```python
from build123d import *
from build123d.topology import SkipClean

# Parameters (mm, degrees)
EXTRUDE1_DEPTH               = 0.000254
SKETCH8_R                    = 2.413
EXTRUDE8_DEPTH               = 7.62
SKETCH6_R                    = 5.715
EXTRUDE6_DEPTH               = 2.413
SKETCH4_R                    = 0.254
EXTRUDE4_DEPTH               = 6.731
SKETCH5_R                    = 1.0033
EXTRUDE5_DEPTH               = 12.954
FILLET2_R                    = 0.889
CHAMFER1_SIZE                = 0.635
CHAMFER3_SIZE                = 0.635
EXTRUDE9_DEPTH               = 12.954
EXTRUDE11_DEPTH              = 6.731
CIRPATTERN1_COUNT            = 8
EXTRUDE12_DEPTH              = 6.731
CHAMFER4_SIZE                = 0.381
CHAMFER4_SIZE2               = 0.659911358
EXTRUDE13_DEPTH              = 0.6604
CUT_REVOLVE1_ANGLE           = 130
CUT_REVOLVE1_OTHER_WAY_ANGLE = 90
BOSS_EXTRUDE1_DEPTH          = 6.071088642
CUT_EXTRUDE1_DEPTH           = 0.838688642
CHAMFER5_SIZE                = 0.1016
CHAMFER6_SIZE                = 0.3048
SKETCH27_R                   = 0.381
CUT_EXTRUDE5_DEPTH           = 16.268548261
CUT_EXTRUDE7_DEPTH           = 1.27
SKETCH29_R                   = 0.6604
BOSS_EXTRUDE2_DEPTH          = 1.016
BOSS_EXTRUDE3_START          = -0.762
SKETCH30_R                   = 1.0033
BOSS_EXTRUDE3_DEPTH          = 0.762


with BuildPart() as part:
    # Sketch1 → Extrude1 (new body)
    with BuildSketch(Plane.XY):
        with BuildLine():
            Line((-1.242889362, 3.556), (-1.813523477, 0.319773119))
            ThreePointArc((-1.813523477, 0.319773119), (0, -1.8415), (1.813523477, 0.319773119))
            Line((1.813523477, 0.319773119), (1.242889362, 3.556))
            Line((1.242889362, 3.556), (-1.242889362, 3.556))
        make_face()
    extrude(amount=EXTRUDE1_DEPTH)

    # Sketch8 → Extrude8 (add)
    with BuildSketch(Plane.XY.offset(0.000254)):
        with Locations(Location((0, 0, 0), (0, 0, 129.743387424))):
            Circle(SKETCH8_R)
    extrude(amount=EXTRUDE8_DEPTH)

    # Sketch6 → Extrude6 (add)
    with BuildSketch(Plane.XY.offset(0.000254)):
        Circle(SKETCH6_R)
    extrude(amount=EXTRUDE6_DEPTH)

    # Sketch4 → Extrude4 (cut)
    with BuildSketch(Plane.XY.offset(7.620254)):
        Circle(SKETCH4_R)
    extrude(amount=-EXTRUDE4_DEPTH, mode=Mode.SUBTRACT)

    # Sketch5 → Extrude5 (add)
    with BuildSketch(Plane(origin=(0, 0, 0), x_dir=(-1, 0, 0), z_dir=(0, 0, -1))):
        with Locations(Location((0, 0, 0), (0, 0, 180))):
            Circle(SKETCH5_R)
    extrude(amount=EXTRUDE5_DEPTH)

    # Fillet2
    fillet2_edges = [part.edges().sort_by_distance(p)[0] for p in [
        (1.242889362, 3.556, 0.000127),
        (-1.242889362, 3.556, 0.000127),
    ]]
    fillet(fillet2_edges, radius=FILLET2_R)

    # Chamfer1
    chamfer1_edges = [part.edges().sort_by_distance(p)[0] for p in [
        (-5.715, 0, 0.000254),
    ]]
    chamfer(chamfer1_edges, length=CHAMFER1_SIZE)

    # Chamfer3
    chamfer3_edges = [part.edges().sort_by_distance(p)[0] for p in [
        (-5.715, 0, 2.413254),
    ]]
    chamfer(chamfer3_edges, length=CHAMFER3_SIZE)

    # Sketch9 → Extrude9 (add)
    with BuildSketch(Plane(origin=(0, 0, 0), x_dir=(-1, 0, 0), z_dir=(0, 0, -1))):
        with BuildLine():
            Line((-0.3175, 3.302), (0.3175, 3.302))
            ThreePointArc((0.3175, 3.302), (0.586907684, 3.190407684), (0.6985, 2.921))
            Line((0.6985, 2.921), (0.6985, 0))
            Line((0.6985, 0), (-0.6985, 0))
            Line((-0.6985, 0), (-0.6985, 2.921))
            ThreePointArc((-0.6985, 2.921), (-0.586907684, 3.190407684), (-0.3175, 3.302))
        make_face()
    extrude(amount=EXTRUDE9_DEPTH)

    # Sketch17 → Extrude11 (cut)
    with BuildSketch(Plane.XY.offset(7.620254)):
        with BuildLine():
            Line((0, 0), (0, 0.8128))
            ThreePointArc((0, 0.8128), (0.077181384, 0.80912723), (0.153665255, 0.798142111))
            ThreePointArc((0.153665255, 0.798142111), (0.281884616, 0.680529664), (0.455713955, 0.673029443))
            ThreePointArc((0.455713955, 0.673029443), (0.517563871, 0.626714831), (0.574736392, 0.574736392))
            Line((0.574736392, 0.574736392), (0, 0))
        make_face()
    extrude11 = extrude(amount=-EXTRUDE11_DEPTH, mode=Mode.SUBTRACT)

    # CirPattern1: Extrude11 ×8 about axis
    cirpattern1_axis = Axis((0, 0, 0), (0, 0, 1))
    for i in range(1, CIRPATTERN1_COUNT):
        add(extrude11.rotate(cirpattern1_axis, i * 360 / CIRPATTERN1_COUNT), mode=Mode.SUBTRACT)

    # Sketch18 → Extrude12 (add)
    with BuildSketch(Plane.XY.offset(7.620254)):
        Polygon((-0.539167209, 0.608229037), (0.811331666, 0.048834087), (0.986294531, 0.471231809), (-0.364204343, 1.030626759), align=None)
    extrude(amount=-EXTRUDE12_DEPTH)

    # Chamfer4
    chamfer4_edges = [part.edges().sort_by_distance(p)[0] for p in [
        (0.136082229, 0.328531562, 7.620254),
    ]]
    chamfer4_side = [part.faces().sort_by_distance(p)[0] for p in [
        (1.499116567, -1.802914954, 7.620254),
    ]]
    chamfer(chamfer4_edges, length=CHAMFER4_SIZE, length2=CHAMFER4_SIZE2, reference=chamfer4_side[0])

    # Sketch19 → Extrude13 (cut)
    with SkipClean():  # the faces are left unmerged after this step: merging them gives an invalid solid
        with BuildSketch(Plane.XY.offset(7.620254)):
            with BuildLine():
                Line((0.811331666, 0.048834087), (-0.539167209, 0.608229037))
                ThreePointArc((-0.539167209, 0.608229037), (-0.311045094, -0.750929284), (0.811331666, 0.048834087))
            make_face()
        extrude(amount=-EXTRUDE13_DEPTH, mode=Mode.SUBTRACT)

    # Sketch20 → Cut-Revolve1 (revolve, cut)
    with SkipClean():  # the faces are left unmerged after this step: merging them gives an invalid solid
        with BuildSketch(Plane(origin=(0, 0, 0), x_dir=(0, 0, -1), z_dir=(1, 0, 0))):
            Polygon((-6.959854, -0.8128), (-6.959854, 0), (-6.147054, 0), align=None)
        revolve(axis=Axis((0, 0, 7.389643883), (0, 0, -1)), revolution_arc=CUT_REVOLVE1_ANGLE, mode=Mode.SUBTRACT)

    # Sketch20 → Cut-Revolve1 other way (revolve, cut)
    with SkipClean():  # the faces are left unmerged after this step: merging them gives an invalid solid
        with BuildSketch(Plane(origin=(0, 0, 0), x_dir=(0, 0, -1), z_dir=(1, 0, 0))):
            Polygon((-6.959854, -0.8128), (-6.959854, 0), (-6.147054, 0), align=None)
        revolve(axis=Axis((0, 0, 7.389643883), (0, 0, 1)), revolution_arc=CUT_REVOLVE1_OTHER_WAY_ANGLE, mode=Mode.SUBTRACT)

    # Sketch21 → Boss-Extrude1 (add)
    with SkipClean():  # the faces are left unmerged after this step: merging them gives an invalid solid
        with BuildSketch(Plane.XY.offset(6.960342642)):
            with BuildLine():
                Line((-0.459893976, 0.575392988), (-0.539167209, 0.608229037))
                ThreePointArc((-0.539167209, 0.608229037), (-0.311045094, -0.750929284), (0.811331666, 0.048834087))
                Line((0.811331666, 0.048834087), (0.732058433, 0.081670135))
                ThreePointArc((0.732058433, 0.081670135), (-0.281884616, -0.680529664), (-0.459893976, 0.575392988))
            make_face()
        extrude(amount=-BOSS_EXTRUDE1_DEPTH)

    # Sketch22 → Cut-Extrude1 (cut)
    with SkipClean():  # the faces are left unmerged after this step: merging them gives an invalid solid
        with BuildSketch(Plane.XY.offset(6.960342642)):
            with BuildLine():
                Line((-0.459893976, 0.575392988), (-0.539167209, 0.608229037))
                ThreePointArc((-0.539167209, 0.608229037), (-0.311045094, -0.750929284), (0.811331666, 0.048834087))
                Line((0.811331666, 0.048834087), (0.732058433, 0.081670135))
                ThreePointArc((0.732058433, 0.081670135), (-0.281884616, -0.680529664), (-0.459893976, 0.575392988))
            make_face()
        extrude(amount=-CUT_EXTRUDE1_DEPTH, mode=Mode.SUBTRACT)

    # Chamfer5
    # the kernel refuses this chamfer: 0.1016 mm, written as the material it takes off along each edge
    with BuildSketch(Plane(origin=(0, 0, 6.121654), x_dir=(-0.3826834323650876, -0.9238795325112875, 0), z_dir=(0.9238795325112875, -0.3826834323650876, 0))) as chamfer5_piece_1_section:
        Polygon((0.7366 + CHAMFER5_SIZE, 0), (0.7366, CHAMFER5_SIZE), (0.7366, 0), align=None)
    chamfer5_piece_1 = revolve(axis=Axis((0, 0, 6.121654), (0, 0, -1)), revolution_arc=45, mode=Mode.PRIVATE)
    chamfer5_piece_1 = chamfer5_piece_1 & Plane(origin=(0, 0, 6.086219336), x_dir=(-0.6633454831704748, 0.74831328329606, 0), z_dir=(0, 0, 1)) * Cylinder(0.8128, 4, mode=Mode.PRIVATE)
    add(chamfer5_piece_1, mode=Mode.SUBTRACT)
    with BuildSketch(Plane(origin=(0, 0, 6.121654), x_dir=(0.3826834323650712, -0.9238795325112945, 0), z_dir=(0.9238795325112945, 0.3826834323650712, 0))) as chamfer5_piece_2_section:
        Polygon((0.7366 + CHAMFER5_SIZE, 0), (0.7366, CHAMFER5_SIZE), (0.7366, 0), align=None)
    chamfer5_piece_2 = revolve(axis=Axis((0, 0, 6.121654), (0, 0, -1)), revolution_arc=45, mode=Mode.PRIVATE)
    chamfer5_piece_2 = chamfer5_piece_2 & Plane(origin=(0, 0, 6.086219336), x_dir=(-0.6633454831704748, 0.74831328329606, 0), z_dir=(0, 0, 1)) * Cylinder(0.8128, 4, mode=Mode.PRIVATE)
    add(chamfer5_piece_2, mode=Mode.SUBTRACT)
    with BuildSketch(Plane(origin=(0, 0, 6.121654), x_dir=(-0.9238795325112938, -0.3826834323650728, 0), z_dir=(0.3826834323650728, -0.9238795325112938, 0))) as chamfer5_piece_3_section:
        Polygon((0.7366 + CHAMFER5_SIZE, 0), (0.7366, CHAMFER5_SIZE), (0.7366, 0), align=None)
    chamfer5_piece_3 = revolve(axis=Axis((0, 0, 6.121654), (0, 0, -1)), revolution_arc=45, mode=Mode.PRIVATE)
    chamfer5_piece_3 = chamfer5_piece_3 & Plane(origin=(0, 0, 6.086219336), x_dir=(-0.6633454831704748, 0.74831328329606, 0), z_dir=(0, 0, 1)) * Cylinder(0.8128, 4, mode=Mode.PRIVATE)
    add(chamfer5_piece_3, mode=Mode.SUBTRACT)
    with BuildSketch(Plane(origin=(0, 0, 6.121654), x_dir=(-0.9238795325112764, 0.3826834323651145, 0), z_dir=(-0.3826834323651145, -0.9238795325112764, 0))) as chamfer5_piece_4_section:
        Polygon((0.7366 + CHAMFER5_SIZE, 0), (0.7366, CHAMFER5_SIZE), (0.7366, 0), align=None)
    chamfer5_piece_4 = revolve(axis=Axis((0, 0, 6.121654), (0, 0, -1)), revolution_arc=49.190233443, mode=Mode.PRIVATE)
    chamfer5_piece_4 = chamfer5_piece_4 & Plane(origin=(0, 0, 6.085867455), x_dir=(-0.6633454831704748, 0.74831328329606, 0), z_dir=(0, 0, 1)) * Cylinder(0.8128, 4, mode=Mode.PRIVATE)
    chamfer5_piece_4 = split(chamfer5_piece_4, bisect_by=Plane(origin=(-0.544175649, 0.610303601, 6.085867455), z_dir=(-0.38268343236508656, -0.9238795325112882, 0)), keep=Keep.TOP, mode=Mode.PRIVATE)
    add(chamfer5_piece_4, mode=Mode.SUBTRACT)
    with BuildSketch(Plane(origin=(0, 0, 6.121654), x_dir=(0.9238795325112772, -0.3826834323651127, 0), z_dir=(0.3826834323651127, 0.9238795325112772, 0))) as chamfer5_piece_5_section:
        Polygon((0.7366 + CHAMFER5_SIZE, 0), (0.7366, CHAMFER5_SIZE), (0.7366, 0), align=None)
    chamfer5_piece_5 = revolve(axis=Axis((0, 0, 6.121654), (0, 0, -1)), revolution_arc=45, mode=Mode.PRIVATE)
    chamfer5_piece_5 = chamfer5_piece_5 & Plane(origin=(0, 0, 6.086219336), x_dir=(-0.6633454831704748, 0.74831328329606, 0), z_dir=(0, 0, 1)) * Cylinder(0.8128, 4, mode=Mode.PRIVATE)
    add(chamfer5_piece_5, mode=Mode.SUBTRACT)
    with BuildSketch(Plane(origin=(0, 0, 6.121654), x_dir=(0.8934479656215565, 0.44916670928142266, 0), z_dir=(-0.44916670928142266, 0.8934479656215565, 0))) as chamfer5_piece_6_section:
        Polygon((0.7366 + CHAMFER5_SIZE, 0), (0.7366, CHAMFER5_SIZE), (0.7366, 0), align=None)
    chamfer5_piece_6 = revolve(axis=Axis((0, 0, 6.121654), (0, 0, -1)), revolution_arc=49.190233443, mode=Mode.PRIVATE)
    chamfer5_piece_6 = chamfer5_piece_6 & Plane(origin=(0, 0, 6.085867455), x_dir=(-0.6633454831704748, 0.74831328329606, 0), z_dir=(0, 0, 1)) * Cylinder(0.8128, 4, mode=Mode.PRIVATE)
    chamfer5_piece_6 = split(chamfer5_piece_6, bisect_by=Plane(origin=(0.816340106, 0.046759523, 6.085867455), z_dir=(-0.38268343236508556, -0.9238795325112885, 0)), keep=Keep.TOP, mode=Mode.PRIVATE)
    add(chamfer5_piece_6, mode=Mode.SUBTRACT)

    # Chamfer6
    chamfer6_edges = [part.edges().sort_by_distance(p)[0] for p in [
        (-0.311045094, -0.750929284, 7.620254),
    ]]
    chamfer(chamfer6_edges, length=CHAMFER6_SIZE)

    # Sketch27 → Cut-Extrude5 (cut, through all)
    with BuildSketch(Plane.XY):
        with Locations((-4.445, 0)):
            Circle(SKETCH27_R)
    extrude(amount=CUT_EXTRUDE5_DEPTH, mode=Mode.SUBTRACT)

    # Sketch28 → Cut-Extrude7 (cut)
    with BuildSketch(Plane(origin=(0, 0, 0.000254), x_dir=(-1, 0, 0), z_dir=(0, 0, -1))):
        with BuildLine():
            Line((4.445, 1.014677811), (6.190751279, 1.413187392))
            ThreePointArc((6.190751279, 1.413187392), (6.35, 0), (6.190751279, -1.413187392))
            Line((6.190751279, -1.413187392), (4.445, -1.014677811))
            ThreePointArc((4.445, -1.014677811), (3.430322189, 0), (4.445, 1.014677811))
        make_face()
    extrude(amount=-CUT_EXTRUDE7_DEPTH, mode=Mode.SUBTRACT)

    # Sketch29 → Boss-Extrude2 (add)
    with BuildSketch(Plane(origin=(0, 0, -12.954), x_dir=(-1, 0, 0), z_dir=(0, 0, -1))):
        Circle(SKETCH29_R)
    extrude(amount=BOSS_EXTRUDE2_DEPTH)

    # Sketch30 → Boss-Extrude3 (add)
    with BuildSketch(Plane(origin=(0, 0, -13.97), x_dir=(-1, 0, 0), z_dir=(0, 0, -1)).offset(BOSS_EXTRUDE3_START)):
        Circle(SKETCH30_R)
    extrude(amount=BOSS_EXTRUDE3_DEPTH)


solid = part.part
```
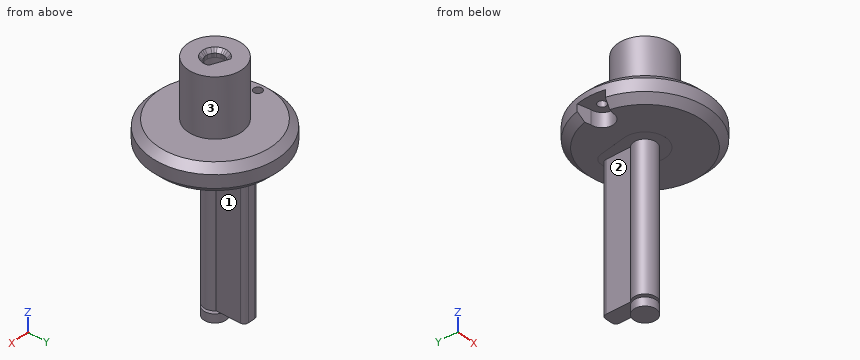
The model under review builds one solid part; all positions refer to its coordinate system, in mm. Face numbers are marked on the shaded views. A direction names the side the tool comes from. Give positions to 0.01 mm unless a question says otherwise; leave off trailing zeros. Write each loop counter-clockwise with the first axis right and the second up, starting at its lowest first coordinate (ties: lowest second). Pieces come first, ordered by that corner, then holes. Notation, with made-up numbers: M 74.25,0.5 L 121.25,0.5 A27 ccw 121.25,16.5 Z; hole C -27.75,18.25 d7. An arc over 180 degrees is marked long. Write item = value, one per line. Start each with the question number.
Q1. For line 1 (X direction, y = 0, z = 1.75) (3 decimals); line 2 (X direction, y = 0, z = 6.3); line 3 (Z direction, x = 4.75, y = -1.75), list the stretches that pass through material, from the lowest coordinate up.
Q2. Clearance check with flat-ended pins moving along their axes: pin 1 (1 mm diameter, centred on x = 1.5, y = 4.5, fed in from +Z); pin 2 (6 mm diameter, centred on x = -1, z = -6.5, fed in from -Y); pin 3 (5 mm diameter, centred on x = -3.5, y = 0.5, fed in from +Z); pin 4 (2.5 mm diameter, centred on y = 1.5, z = -8, fed in from +X). State where each tip first meets the part, or that it passes through.
Q3. We need section B-B (z = -5). State the section outline as (x, y) points, plus the area to 3 significant figures.
Q4. We need section A-A (z = 2). State the section outline as (x, y) points (1 decimal).
Q5. Machinability: for the marked faces 1, 2 and 3, which of the approach directions +Z, -Z, +X, -X, +Y, -Y give a long, thin tool a straight path to every point of the face, cutting with its end or side? Answer none if there is none.
Result set:
q1.line_1 = -5.715 to -4.826, -4.064 to -0.737, 0.737 to 5.715
q1.line_2 = -2.41 to -0.81, 0.81 to 2.41
q1.line_3 = 0 to 2.41
q2.pin_1 = 2.41
q2.pin_2 = -1
q2.pin_3 = 7.62
q2.pin_4 = 0.97
q3.outline = M -0.7,0.72 A1 ccw long 0.7,0.72 L 0.7,2.92 A0.38 ccw 0.32,3.3 L -0.32,3.3 A0.38 ccw -0.7,2.92 Z
q3.area = 6.43 mm2
q4.outline = C 0,0 d11; hole C -4.4,0 d0.8; hole M -0.5,0.6 A0.7 ccw long 0.7,0.1 Z
q5.face_1 = -Z, +X, +Y
q5.face_2 = -Z, -X, +Y
q5.face_3 = +Z
